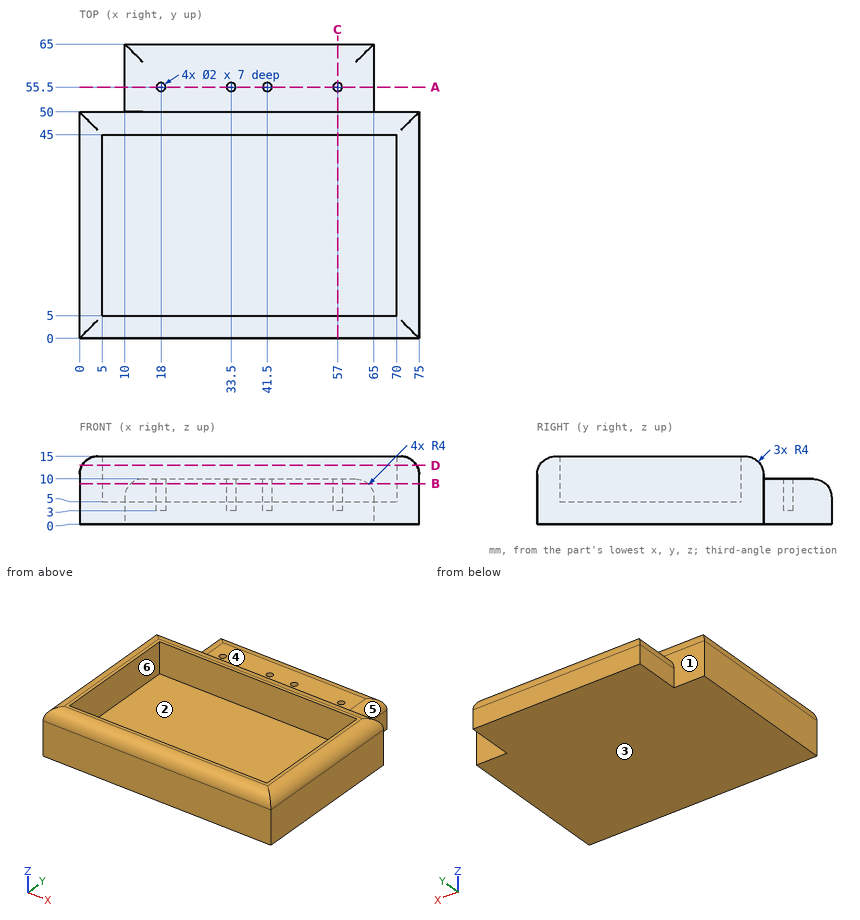
Could you check a few things on this drawing? It's one solid part, dimensions in mm from its lowest x, y, z. A direction names the side the tool comes from. Round coordinates to 2 decimals unless told otherwise and drop trailing zeros. Write each loop counter-clockwise with the first axis right and the second up, starting at its lowest first coordinate (ties: lowest second). Pieces come first, ordered by that corner, then holes. Notation, with made-up numbers: (17.25, 54) -> (51.25, 54) arc R10 ccw to (51.25, 65) -> close; hole circle Ø6 at (18.25, 45). An arc over 180 degrees is marked (long way). Use a Markdown table: item, result.
1. If we section it at D-D (z = 13): List the corners of the cut face in (x, y) for me.
Answer key:
| item | result |
|---|---|
| outline | (0.54, 0.54) -> (74.46, 0.54) -> (74.46, 49.46) -> (0.54, 49.46) -> close; hole (5, 5) -> (70, 5) -> (70, 45) -> (5, 45) -> close |
2. If we section it at B-B (z = 9): List the corners of the cut face in (x, y) for me, then the cut area to 3 significant figures.
Answer key:
| item | result |
|---|---|
| outline | (0, 0) -> (75, 0) -> (75, 50) -> (63.65, 50) -> (63.65, 63.65) -> (11.35, 63.65) -> (11.35, 50) -> (0, 50) -> close; hole (5, 5) -> (70, 5) -> (70, 45) -> (5, 45) -> close; hole circle Ø2 at (18, 55.5); hole circle Ø2 at (33.5, 55.5); hole circle Ø2 at (41.5, 55.5); hole circle Ø2 at (57, 55.5) |
| area | 1,850 mm^2 |
3. If we section it at C-C (x = 57): List the corners of the cut face in (y, z) for me, then the cut area to 3 significant figures.
Answer key:
| item | result |
|---|---|
| outline | (0, 0) -> (65, 0) -> (65, 6) arc R4 ccw to (61, 10) -> (56.5, 10) -> (56.5, 3) -> (54.5, 3) -> (54.5, 10) -> (50, 10) -> (50, 11) arc R4 ccw to (46, 15) -> (45, 15) -> (45, 5) -> (5, 5) -> (5, 15) -> (4, 15) arc R4 ccw to (0, 11) -> close |
| area | 476 mm^2 |
4. For pin 1 Ø3 at (y, z) = (27, 11) entering from -X; pin 2 Ø5 at (x, y) = (45.5, 27) entering from +Z; pin 3 Ø6 at (y, z) = (57.5, 9) entering from +X; pin 4 Ø0.6 at (x, y) = (57, 55.5) entering from +Z, each with a flat end and sliding along its axis, tell me the tip position at first contact or that it passes through.
Answer key:
| item | result |
|---|---|
| pin 1 | stops at x = 0 |
| pin 2 | stops at z = 5 |
| pin 3 | stops at x = 65 |
| pin 4 | stops at z = 3 |
5. We'd pull the mould along Y, two halves only. Please class the marked faces 1, 2 and 3: +Y half, -Y half, draft (parallel to the pull), parting line (faces both ways), or undercut.
Answer key:
| item | result |
|---|---|
| face 1 | +Y half |
| face 2 | undercut |
| face 3 | draft |
6. Which directions (+Z, -Z, +X, -X, +Y, -Y) give clear straight access to the entire face, cutting with the end or side of a thin tool? Please do the marked faces 4, 5 and 6.
Answer key:
| item | result |
|---|---|
| face 4 | +Z, +X, -X, +Y |
| face 5 | +Z, +X, +Y |
| face 6 | +Z |
7. If we section it at A-A (y = 55.5): List the corners of the cut face in (x, z) for me.
Answer key:
| item | result |
|---|---|
| outline | (10, 0) -> (65, 0) -> (65, 6) arc R4 ccw to (61, 10) -> (58, 10) -> (58, 3) -> (56, 3) -> (56, 10) -> (42.5, 10) -> (42.5, 3) -> (40.5, 3) -> (40.5, 10) -> (34.5, 10) -> (34.5, 3) -> (32.5, 3) -> (32.5, 10) -> (19, 10) -> (19, 3) -> (17, 3) -> (17, 10) -> (14, 10) arc R4 ccw to (10, 6) -> close |
8. Please list where these lines run through material, in increasing order: probe 1 along X at (y, z) = (55.5, 5.5); probe 2 along Y at (x, z) = (65.5, 9); probe 3 along Y at (x, z) = (33.5, 8.25).
Answer key:
| item | result |
|---|---|
| probe 1 | x = 10 to 17, 19 to 32.5, 34.5 to 40.5, 42.5 to 56, 58 to 65 |
| probe 2 | y = 0 to 5, 45 to 50 |
| probe 3 | y = 0 to 5, 45 to 54.5, 56.5 to 64.31 |
